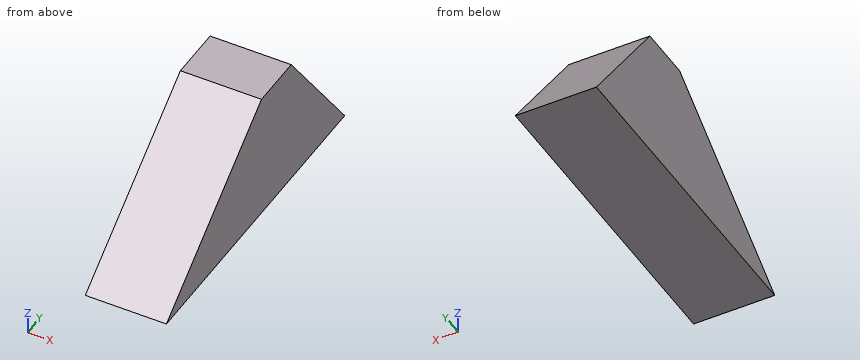
Autodesk Inventor part; units mm, degrees
ref_plane "YZ Plane" through (0, 0, 0) normal (1, 0, 0) x (0, 1, 0)
ref_plane "XZ Plane" through (0, 0, 0) normal (0, 1, 0) x (-1, 0, 0)
ref_plane "XY Plane" through (0, 0, 0) normal (0, 0, 1) x (1, 0, 0)
sketch "Esboço1" plane through (0, 0, 0) normal (0, 1, 0) x (-1, 0, 0)
  line L0 (-12.5, 20) -> (12.5, 20)
  line L1 (12.5, 20) -> (12.5, -20)
  line L2 (12.5, -20) -> (-12.5, -20)
  line L3 (-12.5, -20) -> (-12.5, 20)
  line L4 (-12.5, 20) -> (12.5, -20) construction
  line L5 (12.5, 20) -> (-12.5, -20) construction
  point P0 (0, 0)
  dimension "lenght" = 25
  dimension "widht" = 40
extrude "Extrusão1" add sketch "Esboço1" along normal mid plane 100
sketch "Esboço2" plane through (12.5, -50, -20) normal (1, 0, 0) x (0, 0, -1)
  line L0 (0, 100) -> (0, 0)
  line L1 (0, 100) -> (-40, 70)
  line L2 (-40, 0) -> (-40, 100)
  line L3 (-40, 70) -> (-40, 100)
  line L4 (-40, 100) -> (0, 100)
  point P0 (-20, 50)
  dimension "d4" = 50
extrude "Extrusão2" cut sketch "Esboço2" against normal blind 25
sketch "Esboço3" plane through (12.5, -50, 20) normal (1, 0, 0) x (0, 0, -1)
  line L0 (0, 0) -> (40, 0)
  line L1 (40, 0) -> (0, 53.3331)
  line L2 (0, 70) -> (0, 0)
  line L3 (0, 53.3331) -> (0, 0)
  line L4 (0, 0) -> (40, 0)
  point P0 (20, 50)
  dimension "d7" = 36.87
extrude "Extrusão3" cut sketch "Esboço3" against normal blind 25
equation "\"lenght\" = RIP_L"
equation "\"widht\" = RIP_H"
equation "\"d5\" = RIP_L"
equation "\"d8\" = RIP_L"
equation "\"RIP_H\" = 40"
equation "\"RIP_L\" = 25"
properties part number "feet" material "Madeira"
Geometry: final body of the model. Coordinates: model frame, mm. Give positions to 0.01 mm unless a question says otherwise; leave off trailing zeros. Loops run counter-clockwise (first coordinate to the right, second up) from the corner with the lowest first, then second, coordinate; pieces in that order, holes last. Notation, with made-up numbers: (0, 58.5) - (51, 58.5) arc R24 cw to (51, 80.5) - close; hole circle Ø5 at (-37, -30.5). An arc over 180 degrees is marked (long way). One line per question, with ' | ' between items. Start each with the question number.
(1) Contact query for flat-ended pins moving along their axis: pin 1 (1.5 mm diameter, centred on x = 9.5, z = 4, fed in from -Y); pin 2 (5 mm diameter, centred on x = 8, y = 34, fed in from +Z); pin 3 (3 mm diameter, centred on x = -9.5, z = -13, fed in from -Y). Output: stop coordinate, or through.
(2) Ray query, line 1 (Y direction, x = -5, z = 1.5) (3 decimals); line 2 (Y direction, x = 4.5, z = 5.5) (3 decimals); line 3 (Z direction, x = -10.5, y = 38). Return the intervals inside material, ascending. Write a range as from..to.
(3) Section query A-A on x = 8.75. Return loops of the section in (y, z), then the cut area to 3 significant figures.
(4) Section query B-B on y = 36.5. Return loops of the section in (x, z).
The answers:
1) pin 1: y = -19 | pin 2: z = 4.67 | pin 3: y = -42.67
2) line 1: -21.333..33.875 | line 2: -16..30.875 | line 3: -20..-4
3) outline: (-50, -20) - (50, -20) - (20, 20) - (3.33, 20) - close | area: 2,330 mm2
4) outline: (-12.5, -20) - (12.5, -20) - (12.5, -2) - (-12.5, -2) - close
